For this review, take the finished solid that the model builds, in its own axes (mm). Face numbers are marked on the shaded views. Coordinates: 2 decimals unless noted, no trailing zeros. Loops run counter-clockwise (first coordinate to the right, second up) from the corner with the lowest first, then second, coordinate; pieces in that order, holes last.
1. To check wall thickness, follow probe 1 along Y at (x, z) = (0, 6.75); probe 2 along X at (y, z) = (0, 8.6); probe 3 along X at (y, z) = (-1, 0.5). State the ranges of each line that lie inside material, in increasing order.
2. Clearance check with flat-ended pins moving along their axes: P1, Ø6, axis at x = 0, z = 6, coming from the -Y side; P2, Ø6.5, axis at x = 22.9, y = 39.66, coming from the +Z side; P3, Ø3, axis at y = 45, z = 7.5, coming from the -X side. State where each tip first meets the part, or that it passes through.
3. Mouldability with a two-part tool opening along X and no side actions: class the marked faces 1, 2, 3 and 4 as pulls with the +X half, pulls with the -X half, needs draft (parallel to the pull), parting line crosses it, or undercut.
4. Take a section at B-B, the plane z = 3. Count the separate pieces of the cut face and the enclosed holes in it, then the cut area to 3 significant figures.
5. Take a section at A-A, the plane y = 0. State the section outline as (x, z) points.
6. Take a section at C-C, the plane y = 51. State the section outline as (x, z) points.
7. Take a section at D-D, the plane x = 37. State the section outline as (y, z) points.
Autodesk Inventor part; units mm, degrees
ref_plane "YZ Plane" through (0, 0, 0) normal (1, 0, 0) x (0, 1, 0)
ref_plane "XZ Plane" through (0, 0, 0) normal (0, 1, 0) x (-1, 0, 0)
ref_plane "XY Plane" through (0, 0, 0) normal (0, 0, 1) x (1, 0, 0)
sketch "Sketch1" plane through (0, 0, 0) normal (0, 0, 1) x (1, 0, 0)
  circle A0 centre (0, 0) radius 12.5
  circle A1 centre (-30, 0) radius 3
  circle A2 centre (-15, -25.9808) radius 3
  circle A3 centre (15, -25.9808) radius 3
  circle A4 centre (30, 0) radius 3
  circle A5 centre (15, 25.9808) radius 3
  circle A6 centre (-15, 25.9808) radius 3
  line L0 (0, 57.5) -> (49.7965, 28.75)
  line L1 (49.7965, 28.75) -> (49.7965, -28.75)
  line L2 (49.7965, -28.75) -> (0, -57.5)
  line L3 (0, -57.5) -> (-49.7965, -28.75)
  line L4 (-49.7965, -28.75) -> (-49.7965, 28.75)
  line L5 (-49.7965, 28.75) -> (0, 57.5)
  point P0 (49.7965, 0)
  dimension "d0" = 25
  dimension "d2" = 6
  dimension "d6" = 360
  dimension "d15" = 30
  dimension "d33" = 115
extrude "Extrusion1" add sketch "Sketch1" along normal blind 10 contours A1 | A2 | A3 | A4 | A5 | A6 | L0 L1 L2 L3 L4 L5
sketch "Sketch7" plane through (0, 0, 10) normal (0, 0, 1) x (1, 0, 0)
  circle A0 centre (0, 51) radius 3
  circle A1 centre (-44.1673, 25.5) radius 3
  circle A2 centre (-44.1673, -25.5) radius 3
  circle A3 centre (0, -51) radius 3
  circle A4 centre (44.1673, -25.5) radius 3
  circle A5 centre (44.1673, 25.5) radius 3
  line L0 (0, 51) -> (0, -51)
  point P0 (0, 0)
  dimension "d42" = 6
  dimension "d46" = 360
  dimension "d96" = 102
extrude "Extrusion6" cut sketch "Sketch7" against normal through all
sketch "Sketch9" plane through (0, 0, 0) normal (0, 0, -1) x (-1, 0, 0)
  circle A0 centre (0, 0) radius 25
  dimension "d56" = 50
extrude "Extrusion8" cut sketch "Sketch9" against normal blind 5
sketch "Sketch14" plane through (0, 0, 10) normal (0, 0, 1) x (1, 0, 0)
  circle A0 centre (-45.7965, 0) radius 2.5
  circle A1 centre (-22.8982, -39.6609) radius 2.5
  circle A2 centre (22.8982, -39.6609) radius 2.5
  circle A3 centre (45.7965, 0) radius 2.5
  circle A4 centre (22.8982, 39.6609) radius 2.5
  circle A5 centre (-22.8982, 39.6609) radius 2.5
  line L0 (-49.7965, 28.75) -> (-49.7965, -28.75)
  point P0 (0, 0)
  point P1 (-45.7965, 0)
  dimension "d81" = 5
  dimension "d85" = 360
  dimension "d97" = 4
extrude "Extrusion13" cut sketch "Sketch14" against normal through all
sketch "Sketch15" plane through (0, 0, 10) normal (0, 0, 1) x (1, 0, 0)
  circle A0 centre (-22.8982, 39.6609) radius 2.5
  circle A1 centre (-22.8982, 39.6609) radius 6.5
  circle A2 centre (-45.7965, 0) radius 6.5
  circle A3 centre (-22.8982, -39.6609) radius 6.5
  circle A4 centre (22.8982, -39.6609) radius 6.5
  circle A5 centre (45.7965, 0) radius 6.5
  circle A6 centre (22.8982, 39.6609) radius 6.5
  point P0 (0, 0)
  dimension "d89" = 13
  dimension "d92" = 360
extrude "Extrusion14" cut sketch "Sketch15" against normal blind 5 contours A0 | A1 | A2 | A3 | A4 | A5 | A6
sketch "Sketch16" plane through (0, 0, 5) normal (0, 0, 1) x (1, 0, 0)
  line L0 (-29.3353, 40.5633) -> (-20.4612, 45.6867)
  arc A0 (-29.3353, 40.5633) -> (-20.4612, 45.6867) centre (-22.8982, 39.6609) ccw
  circle A1 centre (-22.8982, 39.6609) radius 2.5
  line L1 (49.7965, 5.1235) -> (49.7965, -5.1235)
  arc A2 (49.7965, 5.1235) -> (49.7965, -5.1235) centre (45.7965, 0) ccw
  circle A3 centre (45.7965, 0) radius 2.5
  line L2 (-20.4612, -45.6867) -> (-29.3353, -40.5633)
  arc A4 (-20.4612, -45.6867) -> (-29.3353, -40.5633) centre (-22.8982, -39.6609) ccw
  circle A5 centre (-22.8982, -39.6609) radius 2.5
  point P0 (0, 0)
extrude "Extrusion15" add sketch "Sketch16" along normal blind 5
sketch "Sketch17" plane through (0, 0, 10) normal (0, 0, 1) x (1, 0, 0)
  circle A0 centre (-22.8982, 39.6609) radius 2.5
  circle A1 centre (45.7965, 0) radius 2.5
  circle A2 centre (-22.8982, -39.6609) radius 2.5
  point P0 (0, 0)
extrude "Extrusion16" add sketch "Sketch17" against normal blind 10
properties part number "TA01" material "ABS Plastic"
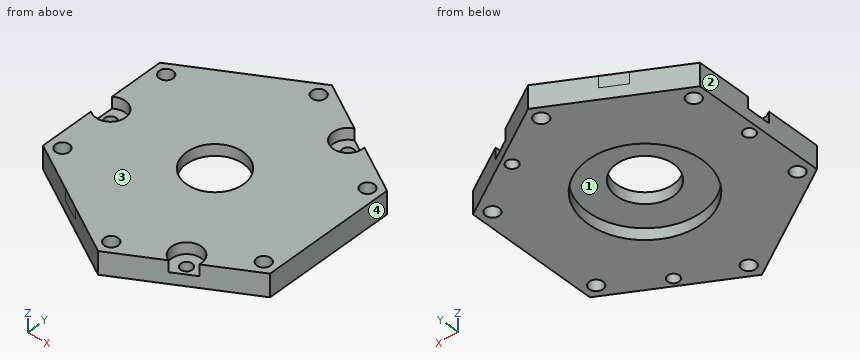
Results list:
1. probe 1: y = -57.5 to -54, -48 to -12.5, 12.5 to 48, 54 to 57.5
1. probe 2: x = -39.3 to -12.5, 12.5 to 49.8
1. probe 3: x = -49.8 to -48.09, -43.51 to -24.98, 24.98 to 49.8
2. P1: stops at y = -57.5
2. P2: stops at z = 5
2. P3: stops at x = -24.25
3. face 1: undercut
3. face 2: pulls with the -X half
3. face 3: needs draft
3. face 4: pulls with the +X half
4. separate pieces: 1
4. enclosed holes: 10
4. area: 6,400 mm2
5. outline: (-49.8, 0) - (-48.3, 0) - (-48.3, 5) - (-49.8, 5) - close; (-43.3, 0) - (-25, 0) - (-25, 5) - (-12.5, 5) - (-12.5, 10) - (-39.3, 10) - (-39.3, 5) - (-43.3, 5) - close; (12.5, 5) - (25, 5) - (25, 0) - (49.8, 0) - (49.8, 10) - (12.5, 10) - close
6. outline: (-11.26, 0) - (-3, 0) - (-3, 10) - (-11.26, 10) - close; (3, 0) - (11.26, 0) - (11.26, 10) - (3, 10) - close
7. outline: (-36.14, 0) - (36.14, 0) - (36.14, 10) - (-36.14, 10) - close
